from build123d import *

# Parameters (mm, degrees)
EXTRUDE_1_DEPTH = 2
SKETCH_2_R      = 7.5
SKETCH_2_R_2    = 3.5
EXTRUDE_2_DEPTH = 2


with BuildPart() as part:
    # 草图1 → 凸台-拉伸1 (new body)
    with BuildSketch(Plane.XY):
        with BuildLine():
            Line((-34.262996942, 15.840978593), (-10.262996942, 15.840978593))
            ThreePointArc((-10.262996942, 15.840978593), (-4.606142692, 13.497832843), (-2.262996942, 7.840978593))
            Line((-2.262996942, 7.840978593), (-2.262996942, -16.159021407))
            ThreePointArc((-2.262996942, -16.159021407), (-4.606142692, -21.815875656), (-10.262996942, -24.159021407))
            Line((-10.262996942, -24.159021407), (-34.262996942, -24.159021407))
            ThreePointArc((-34.262996942, -24.159021407), (-39.919851191, -21.815875656), (-42.262996942, -16.159021407))
            Line((-42.262996942, -16.159021407), (-42.262996942, 7.840978593))
            ThreePointArc((-42.262996942, 7.840978593), (-39.919851191, 13.497832843), (-34.262996942, 15.840978593))
        make_face()
    extrude(amount=EXTRUDE_1_DEPTH)

    # 草图2 → 凸台-拉伸2 (add)
    with BuildSketch(Plane.XY.offset(2)):
        with Locations((-32.472843906, 6.539501993)):
            Circle(SKETCH_2_R)
        with Locations((-32.01907293, -13.566042797)):
            Circle(SKETCH_2_R)
        with Locations((-13.170124689, -4.874583331)):
            Circle(SKETCH_2_R)
        with Locations((-12.925786471, 7.900814922)):
            Circle(SKETCH_2_R_2)
    extrude(amount=EXTRUDE_2_DEPTH)


solid = part.part
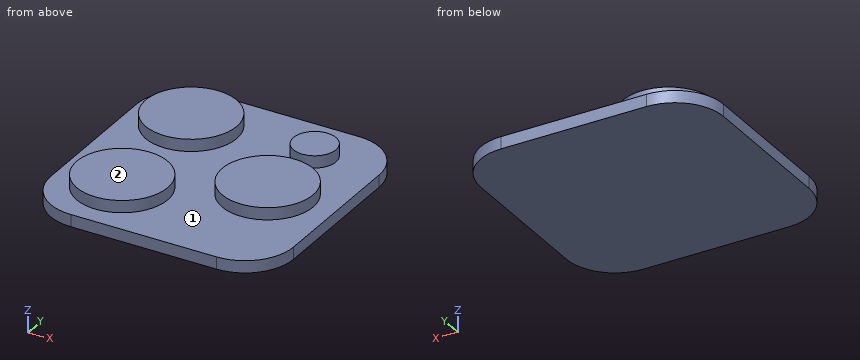
For this review, take the finished solid that the model builds, in its own axes (mm). Face numbers are marked on the shaded views. A direction names the side the tool comes from. Round coordinates to 2 decimals unless told otherwise and drop trailing zeros. Order: outer loops, then holes, each group sorted by start corner. A loop starts at its lowest first (then second) coordinate and runs counter-clockwise, first axis right, second up. Notation, with made-up numbers: (71.5, 36) -> (99.5, 36) arc R22 ccw to (99.5, 48) -> close; hole circle Ø7 at (-20.5, 9.25). An arc over 180 degrees is marked (long way). Write item = value, one per line. Start each with the question number.
1) Take a section at B-B on x = -19. State the section outline as (y, z) points.
2) Take a section at D-D on z = 3.3. State the section outline as (x, y) points, plus the area to 3 significant figures.
3) Take a section at A-A on z = 0.9. State the section outline as (x, y) points, plus the area to 3 significant figures.
4) To check wall thickness, follow line 1 (Z direction, x = -11, y = -17); line 2 (Y direction, x = -32.5, z = 3.1); line 3 (X direction, y = 7, z = 2.5). State the ranges of each line that lie inside material, in increasing order. Write a range as from..to.
5) Tool access review of the marked faces 1 and 2: name each direction out of +Z, -Z, +X, -X, +Y, -Y from which nothing blocks a thin tool from reaching the whole face with its end or side.
6) Take a section at C-C on y = -7. State the section outline as (x, z) points.
Verdict:
q1.outline = (-24.16, 0) -> (15.84, 0) -> (15.84, 2) -> (-0.16, 2) -> (-0.16, 4) -> (-9.59, 4) -> (-9.59, 2) -> (-24.16, 2) -> close
q2.outline = circle Ø15 at (-32.47, 6.54); circle Ø15 at (-32.02, -13.57); circle Ø15 at (-13.17, -4.87); circle Ø7 at (-12.93, 7.9)
q2.area = 569 mm2
q3.outline = (-42.26, -16.16) arc R8 ccw to (-34.26, -24.16) -> (-10.26, -24.16) arc R8 ccw to (-2.26, -16.16) -> (-2.26, 7.84) arc R8 ccw to (-10.26, 15.84) -> (-34.26, 15.84) arc R8 ccw to (-42.26, 7.84) -> close
q3.area = 1,550 mm2
q4.line_1 = 0..2
q4.line_2 = -21.05..-6.08, -0.96..14.04
q4.line_3 = -39.96..-24.99, -16.31..-9.54
q5.face_1 = +Z
q5.face_2 = +Z, +X, -X, +Y, -Y
q6.outline = (-42.26, 0) -> (-2.26, 0) -> (-2.26, 2) -> (-5.98, 2) -> (-5.98, 4) -> (-20.36, 4) -> (-20.36, 2) -> (-28.39, 2) -> (-28.39, 4) -> (-35.64, 4) -> (-35.64, 2) -> (-42.26, 2) -> close
